from build123d import *

# Parameters (mm, degrees)
SKETCH1_R           = 95.25
SKETCH1_R_2         = 66.675
MAIN_ROTOR_DEPTH    = 4.7625
SKETCH2_R           = 2.38125
CUT_SLOTS_DEPTH     = 135.788005424
BOSS_EXTRUDE2_START = -4.7625
SKETCH3_R           = 6.35
BOSS_EXTRUDE2_DEPTH = 4.7625
SKETCH4_R           = 1.27
CUT_EXTRUDE2_DEPTH  = 135.788005424


with BuildPart() as part:
    # Sketch1 → Main Rotor (new body)
    with BuildSketch(Plane(origin=(0, 0, 0), x_dir=(0, 0, -1), z_dir=(1, 0, 0))):
        with Locations(Location((0, 0, 0), (0, 0, 180))):
            Circle(SKETCH1_R)
        with Locations(Location((0, 0, 0), (0, 0, 180))):
            Circle(SKETCH1_R_2, mode=Mode.SUBTRACT)
    extrude(amount=MAIN_ROTOR_DEPTH)

    # Sketch2 → Cut Slots (cut, through all)
    with BuildSketch(Plane(origin=(4.7625, 0, 0), x_dir=(0, 0, -1), z_dir=(1, 0, 0))):
        with Locations((-80.045174165, 14.114123881)):
            Circle(SKETCH2_R)
        with Locations((-82.345264359, 29.97122516)):
            Circle(SKETCH2_R)
        with Locations((-70.411168075, 25.627569339)):
            Circle(SKETCH2_R)
        with Locations((-70.39054482, 40.64)):
            Circle(SKETCH2_R)
        with Locations((-67.128474551, 56.327478237)):
            Circle(SKETCH2_R)
        with Locations((-57.399710123, 48.164075594)):
            Circle(SKETCH2_R)
        with Locations((-52.245776915, 62.264092337)):
            Circle(SKETCH2_R)
        with Locations((-87.63, 0)):
            Circle(SKETCH2_R)
        with Locations((-43.815, 75.889806134)):
            Circle(SKETCH2_R)
        with Locations((-37.465, 64.891283506)):
            Circle(SKETCH2_R)
        with Locations((-74.93, 0)):
            Circle(SKETCH2_R)
        with Locations((-27.79939725, 76.378216217)):
            Circle(SKETCH2_R)
        with Locations((-15.216789809, 86.298703396)):
            Circle(SKETCH2_R)
        with Locations((-13.011457953, 73.791644933)):
            Circle(SKETCH2_R)
        with Locations((0, 81.28)):
            Circle(SKETCH2_R)
        with Locations((15.216789809, 86.298703396)):
            Circle(SKETCH2_R)
        with Locations((13.011457953, 73.791644933)):
            Circle(SKETCH2_R)
        with Locations((27.79939725, 76.378216217)):
            Circle(SKETCH2_R)
        with Locations((43.815, 75.889806134)):
            Circle(SKETCH2_R)
        with Locations((37.465, 64.891283506)):
            Circle(SKETCH2_R)
        with Locations((52.245776915, 62.264092337)):
            Circle(SKETCH2_R)
        with Locations((67.128474551, 56.327478237)):
            Circle(SKETCH2_R)
        with Locations((57.399710123, 48.164075594)):
            Circle(SKETCH2_R)
        with Locations((70.39054482, 40.64)):
            Circle(SKETCH2_R)
        with Locations((82.345264359, 29.97122516)):
            Circle(SKETCH2_R)
        with Locations((70.411168075, 25.627569339)):
            Circle(SKETCH2_R)
        with Locations((80.045174165, 14.114123881)):
            Circle(SKETCH2_R)
        with Locations((87.63, 0)):
            Circle(SKETCH2_R)
        with Locations((74.93, 0)):
            Circle(SKETCH2_R)
        with Locations((80.045174165, -14.114123881)):
            Circle(SKETCH2_R)
        with Locations((82.345264359, -29.97122516)):
            Circle(SKETCH2_R)
        with Locations((70.411168075, -25.627569339)):
            Circle(SKETCH2_R)
        with Locations((70.39054482, -40.64)):
            Circle(SKETCH2_R)
        with Locations((67.128474551, -56.327478237)):
            Circle(SKETCH2_R)
        with Locations((57.399710123, -48.164075594)):
            Circle(SKETCH2_R)
        with Locations((52.245776915, -62.264092337)):
            Circle(SKETCH2_R)
        with Locations((43.815, -75.889806134)):
            Circle(SKETCH2_R)
        with Locations((37.465, -64.891283506)):
            Circle(SKETCH2_R)
        with Locations((27.79939725, -76.378216217)):
            Circle(SKETCH2_R)
        with Locations((15.216789809, -86.298703396)):
            Circle(SKETCH2_R)
        with Locations((13.011457953, -73.791644933)):
            Circle(SKETCH2_R)
        with Locations((0, -81.28)):
            Circle(SKETCH2_R)
        with Locations((-15.216789809, -86.298703396)):
            Circle(SKETCH2_R)
        with Locations((-13.011457953, -73.791644933)):
            Circle(SKETCH2_R)
        with Locations((-27.79939725, -76.378216217)):
            Circle(SKETCH2_R)
        with Locations((-43.815, -75.889806134)):
            Circle(SKETCH2_R)
        with Locations((-37.465, -64.891283506)):
            Circle(SKETCH2_R)
        with Locations((-52.245776915, -62.264092337)):
            Circle(SKETCH2_R)
        with Locations((-67.128474551, -56.327478237)):
            Circle(SKETCH2_R)
        with Locations((-57.399710123, -48.164075594)):
            Circle(SKETCH2_R)
        with Locations((-70.39054482, -40.64)):
            Circle(SKETCH2_R)
        with Locations((-82.345264359, -29.97122516)):
            Circle(SKETCH2_R)
        with Locations((-70.411168075, -25.627569339)):
            Circle(SKETCH2_R)
        with Locations((-80.045174165, -14.114123881)):
            Circle(SKETCH2_R)
    extrude(amount=-CUT_SLOTS_DEPTH, mode=Mode.SUBTRACT)

    # Sketch3 → Boss-Extrude2 (add)
    with BuildSketch(Plane(origin=(4.7625, 0, 0), x_dir=(0, 0, -1), z_dir=(1, 0, 0)).offset(BOSS_EXTRUDE2_START)):
        with BuildLine():
            ThreePointArc((15.226370254, -60.56863172), (10.49630902, -58.039692226), (8.604258147, -53.0208121))
            ThreePointArc((8.604258147, -53.0208121), (11.546477683, -42.011879168), (19.60245, -33.952439353))
            ThreePointArc((19.60245, -33.952439353), (30.610115778, -31.005482581), (41.615241134, -33.961912186))
            ThreePointArc((41.615241134, -33.961912186), (45.015693386, -38.109916371), (44.840788615, -43.470739307))
            ThreePointArc((44.840788615, -43.470739307), (40.527102575, -50.964468228), (34.431304095, -57.096768064))
            ThreePointArc((34.431304095, -57.096768064), (57.742243797, -33.3375), (66.662903665, -1.27))
            ThreePointArc((66.662903665, -1.27), (64.400075463, -9.615266258), (60.067158869, -17.097892412))
            ThreePointArc((60.067158869, -17.097892412), (55.512002406, -19.929775856), (50.219499281, -19.058899914))
            ThreePointArc((50.219499281, -19.058899914), (42.156593461, -11.006396586), (39.2049, 0))
            ThreePointArc((39.2049, 0), (42.156593461, 11.006396586), (50.219499281, 19.058899914))
            ThreePointArc((50.219499281, 19.058899914), (55.512002406, 19.929775856), (60.067158869, 17.097892412))
            ThreePointArc((60.067158869, 17.097892412), (64.400075463, 9.615266258), (66.662903665, 1.27))
            ThreePointArc((66.662903665, 1.27), (57.742243797, 33.3375), (34.431304095, 57.096768064))
            ThreePointArc((34.431304095, 57.096768064), (40.527102575, 50.964468228), (44.840788615, 43.470739307))
            ThreePointArc((44.840788615, 43.470739307), (45.015693386, 38.109916371), (41.615241134, 33.961912186))
            ThreePointArc((41.615241134, 33.961912186), (30.610115778, 31.005482581), (19.60245, 33.952439353))
            ThreePointArc((19.60245, 33.952439353), (11.546477683, 42.011879168), (8.604258147, 53.0208121))
            ThreePointArc((8.604258147, 53.0208121), (10.49630902, 58.039692226), (15.226370254, 60.56863172))
            ThreePointArc((15.226370254, 60.56863172), (23.872972888, 60.579734486), (32.23159957, 58.366768064))
            ThreePointArc((32.23159957, 58.366768064), (0, 66.675), (-32.23159957, 58.366768064))
            ThreePointArc((-32.23159957, 58.366768064), (-23.872972888, 60.579734486), (-15.226370254, 60.56863172))
            ThreePointArc((-15.226370254, 60.56863172), (-10.49630902, 58.039692226), (-8.604258147, 53.0208121))
            ThreePointArc((-8.604258147, 53.0208121), (-11.546477683, 42.011879168), (-19.60245, 33.952439353))
            ThreePointArc((-19.60245, 33.952439353), (-30.610115778, 31.005482581), (-41.615241134, 33.961912186))
            ThreePointArc((-41.615241134, 33.961912186), (-45.015693386, 38.109916371), (-44.840788615, 43.470739307))
            ThreePointArc((-44.840788615, 43.470739307), (-40.527102575, 50.964468228), (-34.431304095, 57.096768064))
            ThreePointArc((-34.431304095, 57.096768064), (-57.742243797, 33.3375), (-66.662903665, 1.27))
            ThreePointArc((-66.662903665, 1.27), (-64.400075463, 9.615266258), (-60.067158869, 17.097892412))
            ThreePointArc((-60.067158869, 17.097892412), (-55.512002406, 19.929775856), (-50.219499281, 19.058899914))
            ThreePointArc((-50.219499281, 19.058899914), (-42.156593461, 11.006396586), (-39.2049, 0))
            ThreePointArc((-39.2049, 0), (-42.156593461, -11.006396586), (-50.219499281, -19.058899914))
            ThreePointArc((-50.219499281, -19.058899914), (-55.512002406, -19.929775856), (-60.067158869, -17.097892412))
            ThreePointArc((-60.067158869, -17.097892412), (-64.400075463, -9.615266258), (-66.662903665, -1.27))
            ThreePointArc((-66.662903665, -1.27), (-57.742243797, -33.3375), (-34.431304095, -57.096768064))
            ThreePointArc((-34.431304095, -57.096768064), (-40.527102575, -50.964468228), (-44.840788615, -43.470739307))
            ThreePointArc((-44.840788615, -43.470739307), (-45.015693386, -38.109916371), (-41.615241134, -33.961912186))
            ThreePointArc((-41.615241134, -33.961912186), (-30.610115778, -31.005482581), (-19.60245, -33.952439353))
            ThreePointArc((-19.60245, -33.952439353), (-11.546477683, -42.011879168), (-8.604258147, -53.0208121))
            ThreePointArc((-8.604258147, -53.0208121), (-10.49630902, -58.039692226), (-15.226370254, -60.56863172))
            ThreePointArc((-15.226370254, -60.56863172), (-23.872972888, -60.579734486), (-32.23159957, -58.366768064))
            ThreePointArc((-32.23159957, -58.366768064), (0, -66.675), (32.23159957, -58.366768064))
            ThreePointArc((32.23159957, -58.366768064), (23.872972888, -60.579734486), (15.226370254, -60.56863172))
        make_face()
        Circle(SKETCH3_R, mode=Mode.SUBTRACT)
    extrude(amount=BOSS_EXTRUDE2_DEPTH)

    # Sketch4 → Cut-Extrude2 (cut, through all)
    with BuildSketch(Plane.ZY):
        with Locations((0, 45.212)):
            Circle(SKETCH4_R)
        with Locations((39.154740556, 22.606)):
            Circle(SKETCH4_R)
        with Locations((39.154740556, -22.606)):
            Circle(SKETCH4_R)
        with Locations((0, -45.212)):
            Circle(SKETCH4_R)
        with Locations((-39.154740556, -22.606)):
            Circle(SKETCH4_R)
        with Locations((-39.154740556, 22.606)):
            Circle(SKETCH4_R)
    extrude(amount=-CUT_EXTRUDE2_DEPTH, mode=Mode.SUBTRACT)


solid = part.part
Build history of the part. All positions in model axes, mm. Give positions to 0.01 mm unless a question says otherwise; leave off trailing zeros. Loops run counter-clockwise (first coordinate to the right, second up) from the corner with the lowest first, then second, coordinate; pieces in that order, holes last. Notation, with made-up numbers: (43.5, 47.5) -> (51.5, 47.5) arc R27 ccw to (51.5, 77.5) -> close; hole circle Ø11 at (43.25, -24). An arc over 180 degrees is marked (long way). Answer in a Markdown table with one row per item.
Item 1: Slice it at B-B on y = -40.64. Write the cut outline in (x, z), plus the area to 3 significant figures.
Findings below:
| item | result |
|---|---|
| outline | (0, -86.14) -> (4.76, -86.14) -> (4.76, -72.77) -> (0, -72.77) -> close; (0, -68.01) -> (4.76, -68.01) -> (4.76, -45.42) -> (0, -45.42) -> close; (0, -12.41) -> (4.76, -12.41) -> (4.76, 12.41) -> (0, 12.41) -> close; (0, 45.42) -> (4.76, 45.42) -> (4.76, 68.01) -> (0, 68.01) -> close; (0, 72.77) -> (4.76, 72.77) -> (4.76, 86.14) -> (0, 86.14) -> close |
| area | 461 mm² |
Item 2: Probe line 1 along Y through (x, z) = (1.2, 0); line 2 along Y through (x, z) = (3.9, -82); line 3 along Y through (x, z) = (1.25, -19). List the from-to ranges inside material, lowest first. Write a range as [from, to].
Findings below:
| item | result |
|---|---|
| line 1 | y = [-95.25, -83.66], [-78.9, -46.48], [-43.94, -6.35], [6.35, 43.94], [46.48, 78.9], [83.66, 95.25] |
| line 2 | y = [-48.46, -32.33], [-27.62, -15.47], [-12.75, 12.75], [15.47, 27.62], [32.33, 48.46] |
| line 3 | y = [-93.34, -60.85], [-34.31, 34.31], [60.85, 93.34] |
Item 3: Slice it at C-C on x = 2.7. Give the number of separate pieces and of enclosed holes in the cut face, plus the area to 3 significant figures.
Findings below:
| item | result |
|---|---|
| separate pieces | 1 |
| enclosed holes | 67 |
| area | 22,400 mm² |
Item 4: Flat gauge pins, fed straight in: P1, Ø5, axis at y = -9.5, z = 25.5, coming from the -X side; P2, Ø1, axis at x = 3, y = 27, coming from the +Z side; P3, Ø2, axis at x = 1.5, z = -17, coming from the -Y side. Where does each tip first touch, or does it go through?
Findings below:
| item | result |
|---|---|
| P1 | stops at x = 0 |
| P2 | stops at z = 91.49 |
| P3 | stops at y = -93.9 |
Item 5: Slice it at A-A on y = 81.28. Write the cut outline in (x, z).
Findings below:
| item | result |
|---|---|
| outline | (0, -49.66) -> (4.76, -49.66) -> (4.76, -2.38) -> (0, -2.38) -> close; (0, 2.38) -> (4.76, 2.38) -> (4.76, 49.66) -> (0, 49.66) -> close |
